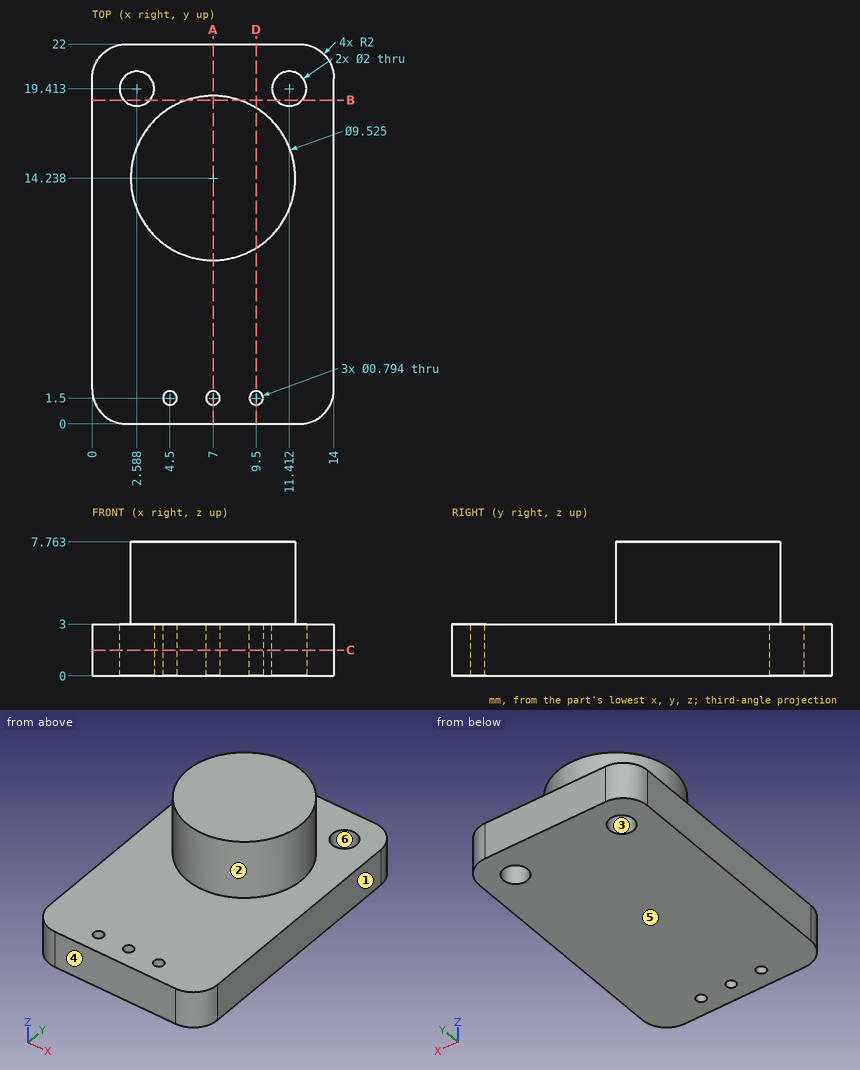
Can you work these out from the drawing? Everything is in mm from the part's minimum corner. A direction names the side the tool comes from. Give positions to 0.01 mm unless a question says otherwise; leave off trailing zeros. Loops run counter-clockwise (first coordinate to the right, second up) from the corner with the lowest first, then second, coordinate; pieces in that order, holes last. Notation, with made-up numbers: M 88,-19.5 L 145,-19.5 A28 cw 145,12.5 Z; hole C -25.75,47 d8. An arc over 180 degrees is marked long. Put each result on its own line as item: value. Start each with the question number.
(1) For the marked faces 1 and 2, which set-ups out of +Z, -Z, +X, -X, +Y, -Y let a thin tool reach every point of the face, with its end or its side?
(2) Will these pins go through, and if not, where does the flat tip stop? pin 1 Ø1.5 at (y, z) = (16.5, 4.5) entering from +X (1 decimal); pin 2 Ø3 at (x, z) = (12.5, 5) entering from +Y (1 decimal); pin 3 Ø1.2 at (x, y) = (11.41, 19.41) entering from +Z; pin 4 Ø4 at (y, z) = (19.5, 6) entering from -X.
(3) I want a section at C-C on z = 1.5. Please give me the cut outline in (x, y), then the cut area to 3 significant figures.
(4) If we mould it in two halves opening along Y, with no side actions, what happens to the marked faces 3, 4, 5 and 6? For each: +Y half, -Y half, draft (parallel to the pull), parting line (faces both ways), or undercut.
(5) I want a section at B-B on y = 18.75. Please give me the cut outline in (x, z).
(6) I want a section at A-A on x = 7. Please give me the cut outline in (y, z) (1 decimal).
(7) I want a section at D-D on x = 9.5. Please give me the cut outline in (y, z).
(8) I need wall thicknesses on line 1 along Y through (x, z) = (4.5, 1.4); line 2 along Z through (x, y) = (12.5, 17.5); line 3 along Y through (x, z) = (6.75, 1). Which ranges of each line are inside material? Lowest first, please. Write a range as [from, to].
Answer block:
1. face 1: +Z, -Z, +X, +Y, -Y
1. face 2: +Z
2. pin 1: x = 11.5
2. pin 2: y = 16.8
2. pin 3: through
2. pin 4: x = 3.53
3. outline: M 0,2 A2 ccw 2,0 L 12,0 A2 ccw 14,2 L 14,20 A2 ccw 12,22 L 2,22 A2 ccw 0,20 Z; hole C 2.59,19.41 d2; hole C 4.5,1.5 d0.79; hole C 7,1.5 d0.79; hole C 9.5,1.5 d0.79; hole C 11.41,19.41 d2
3. area: 297 mm^2
4. face 3: undercut
4. face 4: -Y half
4. face 5: draft
4. face 6: undercut
5. outline: M 0,0 L 1.84,0 L 1.84,3 L 0,3 Z; M 3.34,0 L 10.66,0 L 10.66,3 L 8.52,3 L 8.52,7.76 L 5.48,7.76 L 5.48,3 L 3.34,3 Z; M 12.16,0 L 14,0 L 14,3 L 12.16,3 Z
6. outline: M 0,0 L 1.1,0 L 1.1,3 L 0,3 Z; M 1.9,0 L 22,0 L 22,3 L 19,3 L 19,7.8 L 9.5,7.8 L 9.5,3 L 1.9,3 Z
7. outline: M 0,0 L 1.1,0 L 1.1,3 L 0,3 Z; M 1.9,0 L 22,0 L 22,3 L 18.29,3 L 18.29,7.76 L 10.18,7.76 L 10.18,3 L 1.9,3 Z
8. line 1: [0, 1.1], [1.9, 22]
8. line 2: [0, 3]
8. line 3: [0, 1.19], [1.81, 22]
